```python
from build123d import *

# Parameters (mm, degrees)
F1_W     = 15
F1_H     = 15
F1_W_2   = 13
F1_H_2   = 13
F2_DEPTH = 229
F4_DEPTH = 25


with BuildPart() as f2:
    # F1 (on Top) → F2 (new body)
    with BuildSketch(Plane.XY):
        Rectangle(F1_W, F1_H)
        Rectangle(F1_W_2, F1_H_2, mode=Mode.SUBTRACT)
    extrude(amount=F2_DEPTH)

    # F3 (on face) → F4 (cut)
    with BuildSketch(Plane.XZ.offset(7.5)):
        Polygon((7.5, 0), (-7.5, 15), (-7.5, 0), align=None)
        Polygon((7.5, 229), (-7.5, 229), (-7.5, 214), align=None)
    extrude(amount=-F4_DEPTH, mode=Mode.SUBTRACT)


solid = f2.part
```
Work out the finished part from the listing and answer in its coordinate system (mm). A direction names the side the tool comes from. Round coordinates to 2 decimals unless told otherwise and drop trailing zeros. Write each loop counter-clockwise with the first axis right and the second up, starting at its lowest first coordinate (ties: lowest second). Pieces come first, ordered by that corner, then holes.
1) Determine the mould class of faces 3 (the face through (-7.5, 0, 113)), 4 (the face through (0, 7.5, 113)), 5 (the face through (6.5, 0, 113)), 6 (the face through (0, 6.5, 113)) for opening direction Y: pulls with the +Y half, pulls with the -Y half, needs draft (parallel to the pull), parting line crosses it, or undercut.
2) A cutting plane is placed at B-B on x = -3.75. Determine the outline of the cut face in (y, z).
3) A cutting plane is placed at C-C on z = 180.5. Determine the outline of the cut face in (x, y).
4) Which of the six approach directions +Z, -Z, +X, -X, +Y, -Y give full straight-line access (tool end or side, diameter ignored) to faces 1 (the face through (-0.1, -6.8, 221.4)), 2 (the face through (-6.5, 0, 113))?
5) Consider probe 1 along Y at (x, z) = (-4, 75); probe 2 along Z at (x, y) = (6.75, 6). Determine where each line is inside the solid, lowest interval first.
6) A cutting plane is placed at A-A on y = -2. Determine the outline of the cut face in (x, z), and give its area (3 significant figures).
7) Flat-ended cylindrical pins translate along their axes: P1, Ø4, axis at x = 5, y = 1, coming from the +Z side; P2, Ø8, axis at x = -2, y = 0, coming from the +Z side; P3, Ø5, axis at x = 4.5, y = 2, coming from the -Z side. Find the tip coordinate at first contact, or state that the pin passes through.
Entries:
1. face 3: needs draft
1. face 4: pulls with the +Y half
1. face 5: undercut
1. face 6: undercut
2. outline: (-7.5, 11.25) - (-6.5, 11.25) - (-6.5, 217.75) - (-7.5, 217.75) - close; (6.5, 11.25) - (7.5, 11.25) - (7.5, 217.75) - (6.5, 217.75) - close
3. outline: (-7.5, -7.5) - (7.5, -7.5) - (7.5, 7.5) - (-7.5, 7.5) - close; hole (-6.5, -6.5) - (6.5, -6.5) - (6.5, 6.5) - (-6.5, 6.5) - close
4. face 1: +Z, -X, +Y, -Y
4. face 2: +Z, -Z
5. probe 1: y = -7.5 to -6.5, 6.5 to 7.5
5. probe 2: z = 0.75 to 228.25
6. outline: (-7.5, 15) - (-6.5, 14) - (-6.5, 215) - (-7.5, 214) - close; (6.5, 1) - (7.5, 0) - (7.5, 229) - (6.5, 228) - close
6. area: 428 mm2
7. P1: stops at z = 228.5
7. P2: passes through
7. P3: stops at z = 0.5
